Verification items for the finished model (mm, model axes). A direction names the side the tool comes from. Round coordinates to 2 decimals unless told otherwise and drop trailing zeros. Order: outer loops, then holes, each group sorted by start corner. A loop starts at its lowest first (then second) coordinate and runs counter-clockwise, first axis right, second up. Notation, with made-up numbers: (83, 88) -> (141, 88) arc R20 cw to (141, 126) -> close; hole circle Ø10 at (-27, 56.25). An arc over 180 degrees is marked (long way). Return JSON: item names as keys, results as strings. Group by question number.
Item 1: Scan lines: probe 1 along Z at (x, y) = (3.5, 1); probe 2 along Y at (x, z) = (-3, 8). Record each from-to range of solid material in increasing order. Write a range as from..to.
Item 2: Draft check along X on faces 1 (the cylindrical face through (-1.54, 1.18, 6.26)), 2 (the flat face through (0, -19.05, 7)), 3 (the flat face through (-19.05, 0, 7)). Enter one of: pulls with the +X half, pulls with the -X half, needs draft (parallel to the pull), parting line crosses it, or undercut.
Item 3: Depth check by flat-ended pin: pin 1 Ø10 at (x, y) = (3.5, -5) entering from +Z. Enter the tip coordinate at first touch or a pass-through.
Item 4: Sectioned sample at A-A on z = 6.75. Record the cut outline in (x, y), plus the area to 3 significant figures.
Item 5: Sectioned sample at B-B on y = 4.5. Record the cut outline in (x, z).
Item 6: Access from +Z, -Z, +X, -X, +Y, -Y to the whole of each face (thin tool, end or side, straight path). Record for faces 4 (the cylindrical face through (0.534, -0.168, 19.032)), 5 (the flat face through (0, 12.827, 6)), 6 (the flat face through (0, 0, -5.08)).
Item 7: Sectioned sample at D-D on x = 0. Record the cut outline in (y, z), plus the area to 3 significant figures.
```python
from build123d import *

# Parameters (mm, degrees)
F0_W      = 38.1
F0_H      = 38.1
F1_DEPTH  = 12.7
F2_W      = 25.654
F2_H      = 25.654
F3_DEPTH  = 12.7
F4_W      = 38.1
F4_H      = 38.1
F5_DEPTH  = 5.08
F6_W      = 38.1
F6_H      = 38.1
F7_DEPTH  = 5.08
F8_R      = 1.939554
F9_DEPTH  = 22.606
F10_R     = 0.53889
F11_DEPTH = 25.4
F12_R     = 0.560167
F13_DEPTH = 25.4


with BuildPart() as f1:
    # F0 (on Top) → F1 (new body)
    with BuildSketch(Plane.XY):
        Rectangle(F0_W, F0_H)
    extrude(amount=F1_DEPTH)

    # F2 (on Top) → F3 (cut)
    with BuildSketch(Plane.XY):
        Rectangle(F2_W, F2_H)
    extrude(amount=F3_DEPTH, mode=Mode.SUBTRACT)

    # F4 (on face) → F5 (join)
    with BuildSketch(Plane.XY.offset(12.7)):
        Rectangle(F4_W, F4_H)
    extrude(amount=F5_DEPTH)

    # F6 (on face) → F7 (join)
    with BuildSketch(Plane(origin=(0, 0, 0), x_dir=(1, 0, 0), z_dir=(0, 0, -1))):
        Rectangle(F6_W, F6_H)
    extrude(amount=F7_DEPTH)

    # F8 (on face) → F9 (join)
    with BuildSketch(Plane(origin=(0, 0, -5.08), x_dir=(1, 0, 0), z_dir=(0, 0, -1))):
        Circle(F8_R)
    extrude(amount=-F9_DEPTH)

    # F10 (on face) → F11 (cut)
    with BuildSketch(Plane(origin=(0, 0, -5.08), x_dir=(1, 0, 0), z_dir=(0, 0, -1))):
        Circle(F10_R)
    extrude(amount=-F11_DEPTH, mode=Mode.SUBTRACT)

    # F12 (on face) → F13 (join)
    with BuildSketch(Plane(origin=(0, 0, -5.08), x_dir=(1, 0, 0), z_dir=(0, 0, -1))):
        Circle(F12_R)
    extrude(amount=-F13_DEPTH)


solid = f1.part
```
Recorded:
{
 "1": {"probe 1": "-5.08..0, 12.7..17.78", "probe 2": "-19.05..-12.83, 12.83..19.05"},
 "2": {"face 1": "undercut", "face 2": "needs draft", "face 3": "pulls with the -X half"},
 "3": {"pin 1": "z = 17.78"},
 "4": {"outline": "(-19.05, -19.05) -> (19.05, -19.05) -> (19.05, 19.05) -> (-19.05, 19.05) -> close; circle Ø3.88 at (0, 0); hole (-12.83, -12.83) -> (12.83, -12.83) -> (12.83, 12.83) -> (-12.83, 12.83) -> close", "area": "805 mm²"},
 "5": {"outline": "(-19.05, -5.08) -> (19.05, -5.08) -> (19.05, 17.78) -> (-19.05, 17.78) -> close; hole (-12.83, 0) -> (12.83, 0) -> (12.83, 12.7) -> (-12.83, 12.7) -> close"},
 "6": {"face 4": "+Z", "face 5": "none", "face 6": "-Z, +X, -X, +Y, -Y"},
 "7": {"outline": "(-19.05, -5.08) -> (19.05, -5.08) -> (19.05, 17.78) -> (0.56, 17.78) -> (0.56, 20.32) -> (-0.56, 20.32) -> (-0.56, 17.78) -> (-19.05, 17.78) -> close; hole (-12.83, 0) -> (-1.94, 0) -> (-1.94, 12.7) -> (-12.83, 12.7) -> close; hole (1.94, 0) -> (12.83, 0) -> (12.83, 12.7) -> (1.94, 12.7) -> close", "area": "597 mm²"}
}
